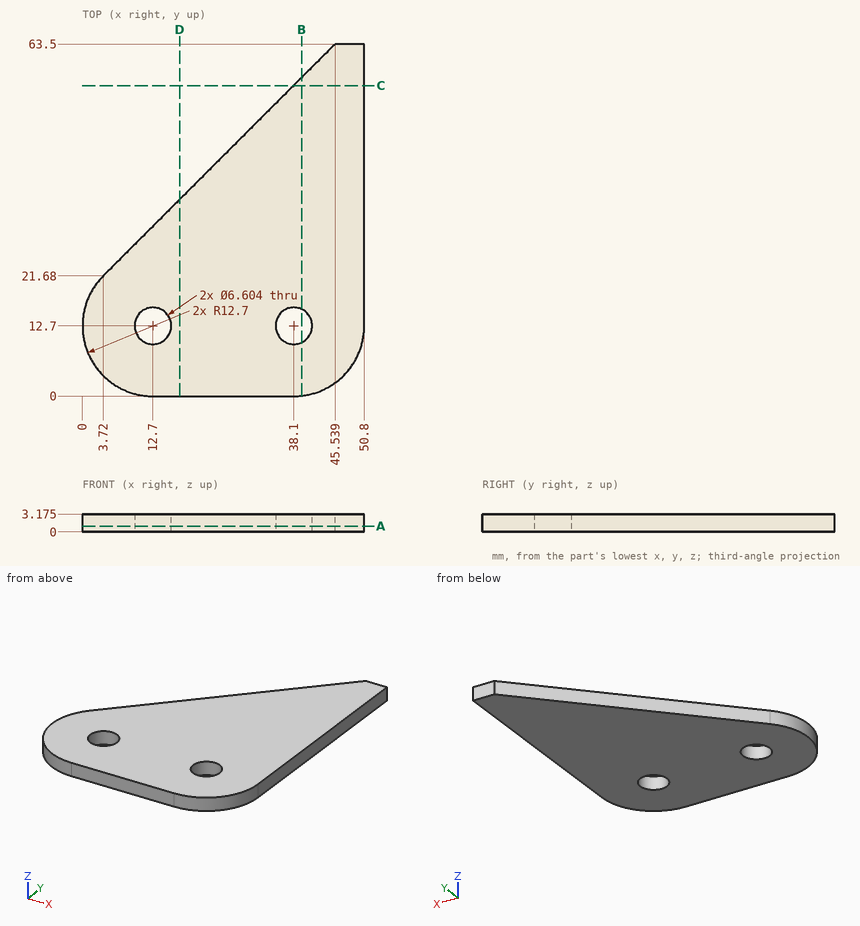
Answer from the drawing. Dimensions are ordinates in mm from the lowest x, y and z of the part. Give positions to 0.01 mm unless a question says otherwise; leave off trailing zeros. Order: outer loops, then holes, each group sorted by start corner. A loop starts at its lowest first (then second) coordinate and runs counter-clockwise, first axis right, second up. Notation, with made-up numbers: (21, 10) -> (60, 10) arc R37 ccw to (60, 47) -> close; hole circle Ø3 at (5.25, 52.5). An arc over 180 degrees is marked (long way). One line per item, written item: value. Start each with the question number.
(1) The part is cut by section D-D (x = 17.5). Determine the outline of the cut face in (y, z) (1 decimal), and give its area (3 significant figures).
(2) Flat-ended cylindrical pins translate along their axes: P1, Ø8.5, axis at x = 38.1, y = 12.7, coming from the -Z side; P2, Ø1.5, axis at y = 41, z = 1, coming from the -X side. Find the tip coordinate at first contact, or state that the pin passes through.
(3) Straight lines are drawn through the part: L1, parallel to X at y = 11.5, z = 1.35 (1 decimal); L2, parallel to Y at x = 37.5, z = 1.65 (1 decimal); L3, parallel to Y at x = 38, z = 1.45. For each, find the intervals that lie inside material, in ascending order.
(4) The part is cut by section B-B (x = 39.5). Determine the outline of the cut face in (y, z) (1 decimal).
(5) The part is cut by section A-A (z = 1.05). Determine the outline of the cut face in (x, y).
(6) The part is cut by section C-C (y = 56). Determine the outline of the cut face in (x, z) (1 decimal).
Taken from the geometry:
1. outline: (0, 0) -> (35.5, 0) -> (35.5, 3.2) -> (0, 3.2) -> close
1. area: 113 mm^2
2. P1: z = 0
2. P2: x = 22.29
3. L1: 0.1 to 9.6, 15.8 to 35, 41.2 to 50.7
3. L2: 0 to 9.5, 15.9 to 55.5
3. L3: 0 to 9.4, 16 to 55.96
4. outline: (0.1, 0) -> (9.7, 0) -> (9.7, 3.2) -> (0.1, 3.2) -> close; (15.7, 0) -> (57.5, 0) -> (57.5, 3.2) -> (15.7, 3.2) -> close
5. outline: (3.72, 21.68) arc R12.7 ccw to (12.7, 0) -> (38.1, 0) arc R12.7 ccw to (50.8, 12.7) -> (50.8, 63.5) -> (45.54, 63.5) -> close; hole circle Ø6.6 at (12.7, 12.7); hole circle Ø6.6 at (38.1, 12.7)
6. outline: (38, 0) -> (50.8, 0) -> (50.8, 3.2) -> (38, 3.2) -> close
